```python
from build123d import *

# Parameters (mm, degrees)
F1_DEPTH = 200
F2_R     = 2
F3_R     = 2


with BuildPart() as f1:
    # F0 (on Front) → F1 (new body)
    with BuildSketch(Plane.XZ):
        with BuildLine():
            ThreePointArc((10, 10), (2.928932, 7.071068), (0, 0))
            Line((0, 0), (120, 0))
            ThreePointArc((120, 0), (117.071068, 7.071068), (110, 10))
            Line((110, 10), (10, 10))
        make_face()
    extrude(amount=F1_DEPTH)

    # F2
    f2_edges = [f1.edges().sort_by_distance(p)[0] for p in [
        (60, -200, 10),
    ]]
    fillet(f2_edges, radius=F2_R)

    # F3
    f3_edges = [f1.edges().sort_by_distance(p)[0] for p in [
        (60, 0, 10),
    ]]
    fillet(f3_edges, radius=F3_R)


solid = f1.part
```
The listing builds one solid part. Answer for the finished solid, in the listing's coordinates (mm). Round coordinates to 2 decimals unless told otherwise and drop trailing zeros. Write each loop counter-clockwise with the first axis right and the second up, starting at its lowest first coordinate (ties: lowest second). Pieces come first, ordered by that corner, then holes. Notation, with made-up numbers: (71.5, 8) -> (77.5, 8) arc R23 cw to (77.5, 47) -> close; hole circle Ø2 at (44, -38). An arc over 180 degrees is marked (long way). Answer as a JSON object with one key per item and string values. Group by question number.
Q1. This flat-tipped pin is pushed along its axis until it touches: pin 1 Ø5 at (x, z) = (89.5, 4) entering from +Y. Where does it stop, or does it pass through?
Q2. Section A-A (y = -44.5) is taken. Write down the section's boundary in (x, z), plus the area to 3 significant figures.
Q3. Determine the mould class of faces 1 (the face through (59, -200, 4)), 2 (the face through (3.01, -98.63, 7.15)), 3 (the face through (117.15, -98.63, 6.99)) for opening direction X: pulls with the +X half, pulls with the -X half, needs draft (parallel to the pull), parting line crosses it, or undercut.
Q4. Straight lines are drawn through the part: line 1 along Z through (x, y) = (115, -97.5); line 2 along X through (y, z) = (-134, 3.5); line 3 along Y through (x, z) = (83, 8.75). For each, find the intervals that lie inside material, in ascending order.
Check values:
{
 "1": {"pin 1": "y = 0"},
 "2": {"outline": "(0, 0) -> (120, 0) arc R10 ccw to (110, 10) -> (10, 10) arc R10 ccw to start", "area": "1,160 mm^2"},
 "3": {"face 1": "needs draft", "face 2": "pulls with the -X half", "face 3": "pulls with the +X half"},
 "4": {"line 1": "0 to 8.66", "line 2": "0.63 to 119.37", "line 3": "-199.85 to -0.15"}
}
